The model under review builds one solid part; all positions refer to its coordinate system, in mm. Coordinates: 2 decimals unless noted, no trailing zeros. Loops run counter-clockwise (first coordinate to the right, second up) from the corner with the lowest first, then second, coordinate; pieces in that order, holes last. Notation, with made-up numbers: M 75.5,48.5 L 124.5,48.5 A21 ccw 124.5,68.5 Z; hole C -29.75,80 d8. An arc over 180 degrees is marked long. Return JSON: item names as keys, results as strings.
```python
from build123d import *

# Parameters (mm, degrees)
BOSS_EXTRUDE1_DEPTH = 31.75
SKETCH2_R           = 1.5875
CUT_EXTRUDE1_DEPTH  = 9.980818595


with BuildPart() as part:
    # Sketch1 → Boss-Extrude1 (new body)
    with BuildSketch(Plane(origin=(0, 0, 0), x_dir=(1, 0, 0), z_dir=(0, 1, 0))):
        with BuildLine():
            Line((-4.7625, 144.4625), (-4.7625, 140.244181405))
            ThreePointArc((-4.7625, 140.244181405), (-15.362391405, 142.792956785), (-25.4, 147.047409447))
            ThreePointArc((-25.4, 147.047409447), (-13.860926819, 148.579861801), (-2.237511623, 149.208224193))
            ThreePointArc((-2.237511623, 149.208224193), (-1.986877125, 149.014193897), (-2.120604202, 148.726822228))
            ThreePointArc((-2.120604202, 148.726822228), (-4.048504895, 146.97068946), (-4.7625, 144.4625))
        make_face()
    extrude(amount=BOSS_EXTRUDE1_DEPTH)

    # Sketch2 → Cut-Extrude1 (cut, through all)
    with BuildSketch(Plane(origin=(0, 0, -149.225), x_dir=(-1, 0, 0), z_dir=(0, 0, -1))):
        with Locations((11.1125, 25.4)):
            Circle(SKETCH2_R)
        with Locations((11.1125, 6.35)):
            Circle(SKETCH2_R)
    extrude(amount=-CUT_EXTRUDE1_DEPTH, mode=Mode.SUBTRACT)


solid = part.part
```
1. The part is to be moulded in two halves that separate along Y. For faces 1 (the face through (-4.762, 16, -142)), 2 (the face through (-11, 31.75, -146)), 3 (the face through (-9.527, 6.42, -145.093)), say which applies: released by +Y, released by -Y, zero draft, split by the parting line, or undercut.
Check values:
{"face 1": "zero draft", "face 2": "released by +Y", "face 3": "undercut"}
2. To check wall thickness, follow line 1 (Y direction, x = -12, z = -143.75); line 2 (X direction, y = 6.35, z = -145.5) (3 decimals); line 3 (Z direction, x = -9.5, y = 14.5). State the ranges of each line that lie inside material, in increasing order.
Check values:
{"line 1": "0 to 5.03, 7.67 to 24.08, 26.72 to 31.75", "line 2": "-22.252 to -12.7, -9.525 to -4.648", "line 3": "-148.92 to -141.16"}
3. Add section D-D on x = -15.75. Give the boundary of the cut face in (y, z).
Check values:
{"outline": "M 0,-148.39 L 31.75,-148.39 L 31.75,-142.92 L 0,-142.92 Z"}
4. Insertion check: pin 1 Ø1 at (y, z) = (20, -147.5) entering from -X; pin 2 Ø1.3 at (y, z) = (23, -142) entering from +X; pin 3 Ø3.5 at (x, y) = (-11.11, 25.4) entering from +Z. Each pin has a flat end and moves straight along its axis. Give the tip position at first contact, or say it passes through.
Check values:
{"pin 1": "x = -25.4", "pin 2": "x = -4.76", "pin 3": "z = -141.12"}
5. Add section B-B on z = -145. State how many separate pieces and enclosed holes the cut face has, plus the area to 3 significant figures.
Check values:
{"separate pieces": "1", "enclosed holes": "2", "area": "505 mm²"}
